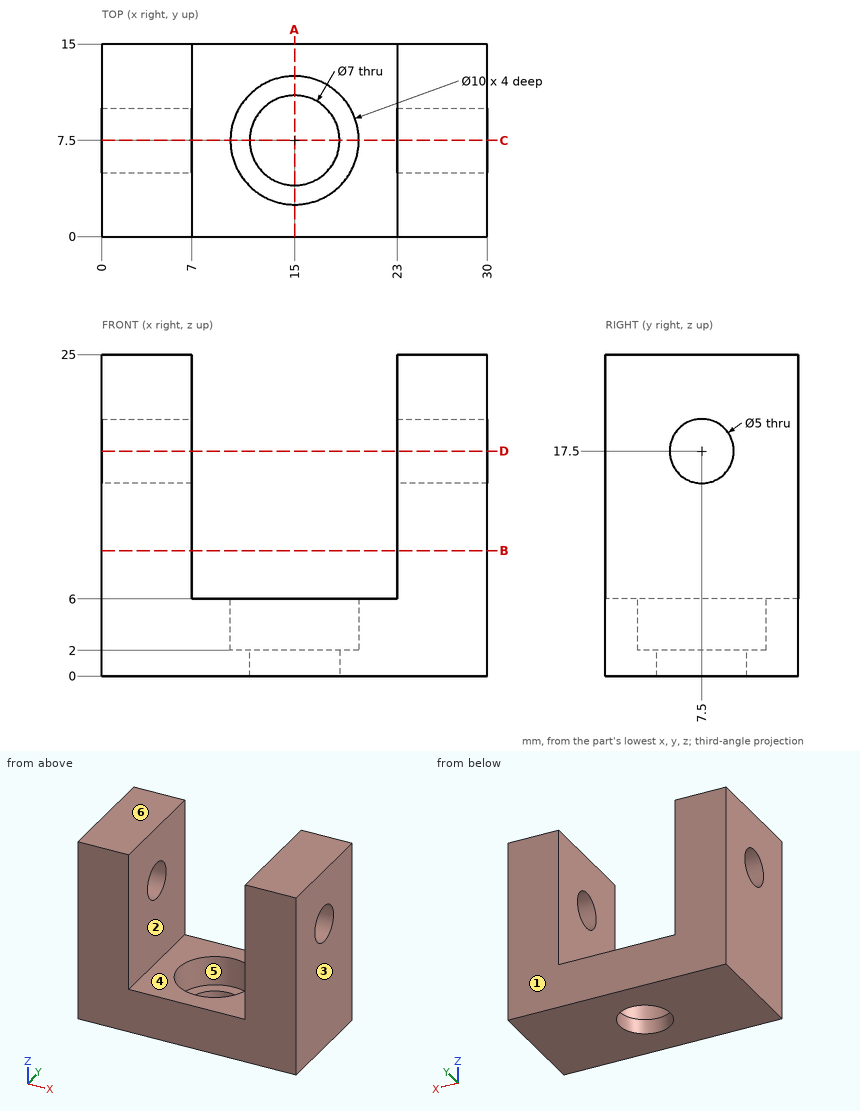
Could you check a few things on this drawing? It's one solid part, dimensions in mm from its lowest x, y, z. A direction names the side the tool comes from. Coordinates: 2 decimals unless noted, no trailing zeros. Order: outer loops, then holes, each group sorted by start corner. A loop starts at its lowest first (then second) coordinate and runs counter-clockwise, first axis right, second up. Notation, with made-up numbers: M -8.75,-39 L 42.25,-39 A11 ccw 42.25,-30 Z; hole C 33,51 d1. An arc over 180 degrees is marked long. Answer as a JSON object with one key per item and string values. Group by question number.
(1) Suppose I cut it at A-A, the plane x = 15. Please give me the cut outline in (y, z).
(2) Suppose I cut it at C-C, the plane y = 7.5. Please give me the cut outline in (x, z).
(3) Which directions (+Z, -Z, +X, -X, +Y, -Y) give clear straight access to the entire face, cutting with the end or side of a thin tool? Please do the marked faces 4, 5 and 6.
(4) If we mould it in two halves opening along X, with no side actions, what happens to the marked faces 1, 2 and 3? For each: released by +X, released by -X, zero draft, split by the parting line, or undercut.
(5) Suppose I cut it at D-D, the plane z = 17.5. Please give me the cut outline in (x, y).
(6) I need wall thicknesses on probe 1 along X at (y, z) = (10.25, 22.75); probe 2 along Y at (x, z) = (26.5, 17.5); probe 3 along Y at (x, z) = (15.25, 1.25). Which ranges of each line are inside material? Lowest first, please.
(7) Suppose I cut it at B-B, the plane z = 9.75. Please give me the cut outline in (x, y), then the cut area to 3 significant figures.
(8) For pin 1 (4.5 mm diameter, centred on x = 16, y = 4.5, fed in from +Z); pin 2 (8 mm diameter, centred on x = 15, y = 7.5, fed in from +Z); pin 3 (3 mm diameter, centred on x = 14.5, y = 6, fed in from +Z), each with a flat end and sliding along its axis, tell me the tip position at first contact or that it passes through.
Values found:
{
 "1": {"outline": "M 0,0 L 4,0 L 4,2 L 2.5,2 L 2.5,6 L 0,6 Z; M 11,0 L 15,0 L 15,6 L 12.5,6 L 12.5,2 L 11,2 Z"},
 "2": {"outline": "M 0,0 L 11.5,0 L 11.5,2 L 10,2 L 10,6 L 7,6 L 7,15 L 0,15 Z; M 0,20 L 7,20 L 7,25 L 0,25 Z; M 18.5,0 L 30,0 L 30,15 L 23,15 L 23,6 L 20,6 L 20,2 L 18.5,2 Z; M 23,20 L 30,20 L 30,25 L 23,25 Z"},
 "3": {"face 4": "+Z, +Y, -Y", "face 5": "+Z", "face 6": "+Z, +X, -X, +Y, -Y"},
 "4": {"face 1": "zero draft", "face 2": "undercut", "face 3": "released by +X"},
 "5": {"outline": "M 0,0 L 7,0 L 7,5 L 0,5 Z; M 0,10 L 7,10 L 7,15 L 0,15 Z; M 23,0 L 30,0 L 30,5 L 23,5 Z; M 23,10 L 30,10 L 30,15 L 23,15 Z"},
 "6": {"probe 1": "x = 0 to 7, 23 to 30", "probe 2": "y = 0 to 5, 10 to 15", "probe 3": "y = 0 to 4.01, 10.99 to 15"},
 "7": {"outline": "M 0,0 L 7,0 L 7,15 L 0,15 Z; M 23,0 L 30,0 L 30,15 L 23,15 Z", "area": "210 mm^2"},
 "8": {"pin 1": "stops at z = 6", "pin 2": "stops at z = 2", "pin 3": "passes through"}
}
